The model under review builds one solid part; all positions refer to its coordinate system, in mm. Round coordinates to 2 decimals unless told otherwise and drop trailing zeros. Order: outer loops, then holes, each group sorted by start corner. A loop starts at its lowest first (then second) coordinate and runs counter-clockwise, first axis right, second up. Notation, with made-up numbers: M 47.5,-2.5 L 88.5,-2.5 A15 cw 88.5,11.5 Z; hole C 42.25,29 d10. An arc over 180 degrees is marked long. Answer as a JSON object with one key per item and string values. Group by question number.
1. To check wall thickness, follow probe 1 along X at (y, z) = (1, 98.5); probe 2 along X at (y, z) = (10, 9.5); probe 3 along Y at (x, z) = (-37.5, 24). State the ranges of each line that lie inside material, in increasing order. Write a range as [from, to].
2. Clearance check with flat-ended pins moving along their axes: P1, Ø2, axis at y = -26.5, z = 44, coming from the +X side; P2, Ø1.5, axis at x = 2.5, y = 0.5, coming from the +Z side; P3, Ø6, axis at y = 18, z = 67.5, coming from the -X side; P4, Ø6, axis at y = 2.5, z = 105, coming from the +X side. State where each tip first meets the part, or that it passes through.
3. Add section A-A on z = 75.5. State the section outline as (x, y) points.
4. Add section B-B on z = 117.5. State the section outline as (x, y) points, and give its area (3 significant figures).
5. Add section D-D on y = 38. State the section outline as (x, z) points.
6. Add section C-C on x = 23. State the section outline as (y, z) points.
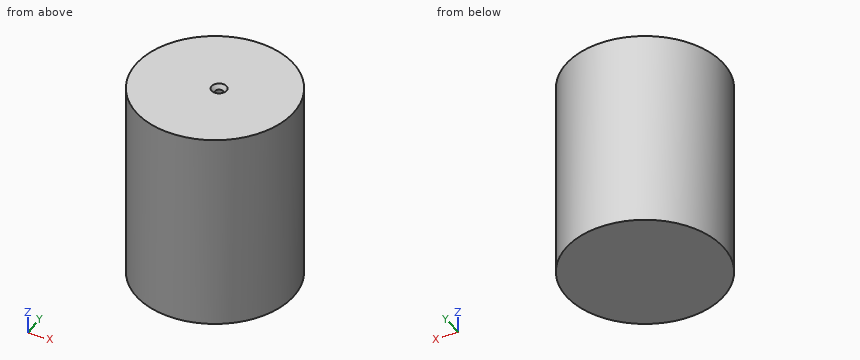
Autodesk Inventor part; units mm, degrees
ref_plane "YZ Plane" through (0, 0, 0) normal (1, 0, 0) x (0, 1, 0)
ref_plane "XZ Plane" through (0, 0, 0) normal (0, 1, 0) x (-1, 0, 0)
ref_plane "XY Plane" through (0, 0, 0) normal (0, 0, 1) x (1, 0, 0)
sketch "Sketch1" plane through (0, 0, 0) normal (0, 0, 1) x (1, 0, 0)
  circle A0 centre (0, 0) radius 50
  dimension "d0" = 100
extrude "Extrusion1" add sketch "Sketch1" along normal blind 127
sketch "Sketch2" plane through (0, 0, 0) normal (0, 0, -1) x (-1, 0, 0)
  point P0 (0, 0)
  point P1 (3.0158, -0.2622)
hole "Hole1" at (-3.0158, -0.2622, 0) direction (0, 0, -1) diameter 5 depth 25.4 tip angle 118
sketch "Sketch3" plane through (0, 0, 127) normal (0, 0, 1) x (1, 0, 0)
  point P0 (0, 0)
  point P1 (2.1463, 0.878)
hole "Hole2" at (2.1463, 0.878, 127) direction (0, 0, -1) diameter 4.9784 depth 19.05 countersink diameter 9.525 countersink angle 82
properties part number "Media container"
Recorded:
{
 "1": {"probe 1": "x = [-49.99, 49.99]", "probe 2": "x = [-48.99, 48.99]", "probe 3": "y = [-33.07, 33.07]"},
 "2": {"P1": "stops at x = 43.01", "P2": "stops at z = 107.95", "P3": "stops at x = -47.7", "P4": "stops at x = 50"},
 "3": {"outline": "C 0,0 d100"},
 "4": {"outline": "C 0,0 d100; hole C 2.15,0.88 d4.98", "area": "7,830 mm²"},
 "5": {"outline": "M -32.5,0 L 32.5,0 L 32.5,127 L -32.5,127 Z"},
 "6": {"outline": "M -44.4,0 L 44.4,0 L 44.4,127 L -44.4,127 Z"}
}
